from build123d import *

# Parameters (mm, degrees)
SKETCH1_R           = 2
SKETCH1_W           = 5.2
SKETCH1_H           = 5.2
BOSS_EXTRUDE1_DEPTH = 5
CONG_1_R            = 15
CONG_2_R            = 3


with BuildPart() as part:
    # Sketch1 → Boss-Extrude1 (new body)
    with BuildSketch(Plane.XY):
        Polygon((24, 5), (9.814954576, 5), (6.350852961, 11), (-6.350852961, 11), (-12.701705922, 0), (-6.350852961, -11), (6.350852961, -11), (9.814954576, -5), (24, -5), (24, -41.569219382), (-48, 0), (24, 41.569219382), align=None)
        with Locations((14, 24.248711306)):
            Circle(SKETCH1_R, mode=Mode.SUBTRACT)
        with Locations((14, -24.248711306)):
            Circle(SKETCH1_R, mode=Mode.SUBTRACT)
        with Locations((-28, 0)):
            Circle(SKETCH1_R, mode=Mode.SUBTRACT)
        with Locations((0, 20.5)):
            Rectangle(SKETCH1_W, SKETCH1_H, mode=Mode.SUBTRACT)
        Polygon((21.305186827, 9.29833395), (16.801854728, 6.69833395), (14.201854728, 11.20166605), (18.705186827, 13.80166605), align=None, mode=Mode.SUBTRACT)
        Polygon((18.705186827, -13.80166605), (14.201854728, -11.20166605), (16.801854728, -6.69833395), (21.305186827, -9.29833395), align=None, mode=Mode.SUBTRACT)
        with Locations((0, -20.5)):
            Rectangle(SKETCH1_W, SKETCH1_H, mode=Mode.SUBTRACT)
        Polygon((-21.305186827, -9.29833395), (-16.801854728, -6.69833395), (-14.201854728, -11.20166605), (-18.705186827, -13.80166605), align=None, mode=Mode.SUBTRACT)
        Polygon((-18.705186827, 13.80166605), (-14.201854728, 11.20166605), (-16.801854728, 6.69833395), (-21.305186827, 9.29833395), align=None, mode=Mode.SUBTRACT)
    extrude(amount=BOSS_EXTRUDE1_DEPTH)

    # Congé1
    cong_1_edges = [part.edges().sort_by_distance(p)[0] for p in [
        (24, -41.569219382, 2.5),
        (-48, 0, 2.5),
        (24, 41.569219382, 2.5),
    ]]
    fillet(cong_1_edges, radius=CONG_1_R)

    # Congé2
    cong_2_edges = [part.edges().sort_by_distance(p)[0] for p in [
        (24, 5, 2.5),
        (9.814954576, 5, 2.5),
        (9.814954576, -5, 2.5),
        (24, -5, 2.5),
    ]]
    fillet(cong_2_edges, radius=CONG_2_R)


solid = part.part
Verification items for the finished model (mm, model axes). A direction names the side the tool comes from. Coordinates: 2 decimals unless noted, no trailing zeros. Write each loop counter-clockwise with the first axis right and the second up, starting at its lowest first coordinate (ties: lowest second). Pieces come first, ordered by that corner, then holes. Notation, with made-up numbers: M 26,8.25 L 54,8.25 A26 ccw 54,41.25 Z; hole C 25.5,65 d3. An arc over 180 degrees is marked long. Use CSV: the item, a comma, the result in double quotes.
Q1. Thickness scan on line 1 along Y through (x, z) = (0, 2.25); line 2 along Y through (x, z) = (14, 2.3); line 3 along X through (y, z) = (13, 1.2). Record the ranges inside material, lowest first. Write a range as [from, to].
Computed values:
line 1,"[-27.71, -23.1], [-17.9, -11], [11, 17.9], [23.1, 27.71]"
line 2,"[-29.73, -26.25], [-22.25, -5], [5, 22.25], [26.25, 29.73]"
line 3,"[-25.48, -19.17], [-17.32, 17.32], [19.17, 24]"
Q2. Mould release check, pull along X, two halves, no side actions. Record for faces 1 (the flat face through (-12.189, 20.675, 2.465)), 2 (the flat face through (-2.6, 20, 2)), 3 (the flat face through (16, 5, 2)): pulls with the +X half, pulls with the -X half, needs draft (parallel to the pull), parting line crosses it, or undercut.
Computed values:
face 1,"pulls with the -X half"
face 2,"undercut"
face 3,"needs draft"
Q3. Section check A-A, the plane x = -16. Enter the section's corners in (y, z).
Computed values:
outline,"M -18.48,0 L -12.24,0 L -12.24,5 L -18.48,5 Z; M -8.09,0 L 8.09,0 L 8.09,5 L -8.09,5 Z; M 12.24,0 L 18.48,0 L 18.48,5 L 12.24,5 Z"
Q4. Section check D-D, the plane z = 2.65. State how many separate pieces and enclosed holes the cut face has, and give its area (3 significant figures).
Computed values:
separate pieces,"1"
enclosed holes,"9"
area,"1,780 mm²"
Q5. Set-up check for faces 4 (the flat face through (0, -11, 2)), 5 (the flat face through (9, 7, 0)), 6 (the flat face through (16, -5, 2)): record each of +Z, -Z, +X, -X, +Y, -Y from which the full face is reachable in a straight line by a thin tool's end or side.
Computed values:
face 4,"+Z, -Z"
face 5,"-Z, +X, -X, +Y, -Y"
face 6,"+Z, -Z, +X"
Q6. Section check B-B, the plane y = -25. Enter the section's corners in (x, z).
Computed values:
outline,"M -4.7,0 L 12.15,0 L 12.15,5 L -4.7,5 Z; M 15.85,0 L 20.68,0 L 20.68,5 L 15.85,5 Z"
Q7. Section check C-C, the plane x = -28. Enter the section's corners in (y, z), and give its area (3 significant figures).
Computed values:
outline,"M -11.18,0 L -2,0 L -2,5 L -11.18,5 Z; M 2,0 L 11.18,0 L 11.18,5 L 2,5 Z"
area,"91.8 mm²"
Q8. Go/stop test with flat-tipped pins: P1, Ø3, axis at x = -25, z = 0.5, coming from the -Y side; P2, Ø1.5, axis at x = 0, z = 2, coming from the +Y side; P3, Ø3, axis at x = -25.5, z = 2.5, coming from the +Y side. Record where each tip stops, or that it passes through.
Computed values:
P1,"y = -14.15"
P2,"y = 28.15"
P3,"y = 13.86"
